Here's how the part is built. I have some questions about the finished solid (model axes, mm). Face numbers are marked on the shaded views. A direction names the side the tool comes from. Round coordinates to 2 decimals unless told otherwise and drop trailing zeros. Write each loop counter-clockwise with the first axis right and the second up, starting at its lowest first coordinate (ties: lowest second). Pieces come first, ordered by that corner, then holes. Notation, with made-up numbers: (1, 24) -> (10, 24) arc R28 ccw to (10, 50) -> close; hole circle Ø9 at (87.5, -30.75). An arc over 180 degrees is marked (long way). Put each result on its own line as item: value. Start each with the question number.
1. We'd pull the mould along Y, two halves only. Please class the marked faces 1, 2 and 3: +Y half, -Y half, draft (parallel to the pull), parting line (faces both ways), or undercut.
2. Suppose I cut it at A-A (x = 18.5). Please give me the cut outline in (y, z), then the cut area to 3 significant figures.
3. I need wall thicknesses on probe 1 along X at (y, z) = (6, -6); probe 2 along Y at (x, z) = (-20, 36); probe 3 along X at (y, z) = (-45.6, 30). Which ranges of each line are inside material? Lowest first, please. Write a range as from..to.
4. For pin 1 (5 mm diameter, centred on x = -20.5, y = -35, fed in from -Z); pin 2 (6.5 mm diameter, centred on x = 0, z = 30, fed in from -Y), each with a flat end and sliding along its axis, tell me the tip position at first contact or that it passes through.
5. Suppose I cut it at C-C (x = 43). Please give me the cut outline in (y, z).
6. Suppose I cut it at B-B (y = 28.5). Please give me the cut outline in (x, z).
7. Suppose I cut it at D-D (z = -34). Please give me the cut outline in (x, y).
8. Which directions (+Z, -Z, +X, -X, +Y, -Y) give clear straight access to the entire face, cutting with the end or side of a thin tool? Please do the marked faces 4 and 5.
```python
from build123d import *

# Parameters (mm, degrees)
F0_W          = 110
F0_H          = 90
F1_DEPTH      = 75
F2_T          = 3
F4_DEPTH      = 25.4
F6_DEPTH      = 25.4
F6_DEPTH_BACK = 126.746


with BuildPart() as f1:
    # F0 (on Top) → F1 (new body, symmetric)
    with BuildSketch(Plane.XY):
        Rectangle(F0_W, F0_H)
    extrude(amount=F1_DEPTH, both=True)

    # F2
    f2_openings = [f1.faces().sort_by_distance(p)[0] for p in [
        (0, 0, -75),
    ]]
    offset(amount=F2_T, openings=f2_openings, kind=Kind.INTERSECTION)

    # F3 (on face) → F4 (cut)
    with BuildSketch(Plane.XY.offset(78)):
        with BuildLine():
            ThreePointArc((45, -10), (52.0710678119, -7.0710678119), (55, 0))
            ThreePointArc((55, 0), (52.0710678119, 7.0710678119), (45, 10))
            ThreePointArc((45, 10), (37.9289321881, 7.0710678119), (35, 0))
            ThreePointArc((35, 0), (37.9289321881, -7.0710678119), (45, -10))
        make_face()
    extrude(amount=-F4_DEPTH, mode=Mode.SUBTRACT)

    # F5 (on face) → F6 (cut, two sides)
    with BuildSketch(Plane(origin=(0, -45, 0), x_dir=(-1, 0, 0), z_dir=(0, 1, 0))) as f6_sk:
        with BuildLine():
            ThreePointArc((4, 30), (-2.8284271247, 32.8284271247), (0, 26))
            ThreePointArc((0, 26), (2.8284271247, 27.1715728753), (4, 30))
        make_face()
    extrude(amount=-F6_DEPTH, mode=Mode.SUBTRACT)
    extrude(f6_sk.sketch, amount=F6_DEPTH_BACK, mode=Mode.SUBTRACT)


solid = f1.part
```
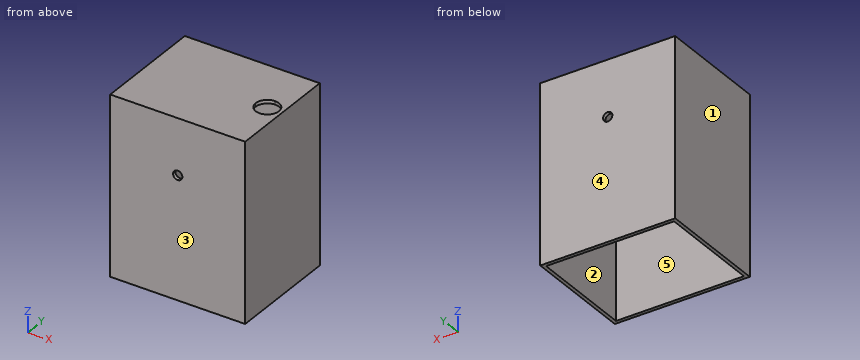
Verdict:
1. face 1: draft
1. face 2: undercut
1. face 3: -Y half
2. outline: (-48, -75) -> (-45, -75) -> (-45, 75) -> (45, 75) -> (45, -75) -> (48, -75) -> (48, 78) -> (-48, 78) -> close
2. area: 1,190 mm^2
3. probe 1: x = -58..-55, 55..58
3. probe 2: y = -48..-45, 45..48
3. probe 3: x = -58..-4, 4..58
4. pin 1: stops at z = 75
4. pin 2: passes through
5. outline: (-48, -75) -> (-45, -75) -> (-45, 75) -> (-9.8, 75) -> (-9.8, 78) -> (-48, 78) -> close; (9.8, 75) -> (45, 75) -> (45, -75) -> (48, -75) -> (48, 78) -> (9.8, 78) -> close
6. outline: (-58, -75) -> (-55, -75) -> (-55, 75) -> (55, 75) -> (55, -75) -> (58, -75) -> (58, 78) -> (-58, 78) -> close
7. outline: (-58, -48) -> (58, -48) -> (58, 48) -> (-58, 48) -> close; hole (-55, -45) -> (55, -45) -> (55, 45) -> (-55, 45) -> close
8. face 4: +Z, -Z, +X, -X, +Y
8. face 5: -Z
